Can you work these out from the model? Positions are in its coordinate system, mm. Give positions to 0.01 mm unless a question says otherwise; leave off trailing zeros. Loops run counter-clockwise (first coordinate to the right, second up) from the corner with the lowest first, then second, coordinate; pieces in that order, holes last. Notation, with made-up numbers: M 75,66.25 L 100,66.25 A20 ccw 100,96.25 Z; hole C -3,63.5 d9. An arc over 180 degrees is marked long. Put each result on its own line as item: value. Start each with the question number.
1) Imagine slicing it at A-A (z = -4). Write out the boundary of the cut face in (x, y).
2) Imagine slicing it at B-B (x = -11). Write out the boundary of the cut face in (y, z), then the cut area to 3 significant figures.
3) Please list where these lines run through material, in increasing order: line 1 along Z through (x, y) = (-44, 2); line 2 along X through (y, z) = (1.55, -50); line 3 along X through (y, z) = (1.35, -7.5). Write a range as from..to.
4) Imagine slicing it at C-C (y = 0.95). State how many separate pieces and enclosed holes the cut face has, then the cut area to 3 significant figures.
from build123d import *

# Parameters (mm, degrees)
SKETCH1_W           = 230
SKETCH1_H           = 103
BOSS_EXTRUDE1_DEPTH = 3
SKETCH2_W           = 85
SKETCH2_H           = 50.2
CUT_EXTRUDE1_DEPTH  = 3
SKETCH3_R           = 1.5
SKETCH3_W           = 31.00355617
SKETCH3_H           = 13
CUT_EXTRUDE2_DEPTH  = 3
SKETCH4_R           = 1
CUT_EXTRUDE3_DEPTH  = 3


with BuildPart() as part:
    # Sketch1 → Boss-Extrude1 (new body)
    with BuildSketch(Plane(origin=(0, 0, 0), x_dir=(1, 0, 0), z_dir=(0, 1, 0))):
        with Locations((2.626404494, 17.846910112)):
            Rectangle(SKETCH1_W, SKETCH1_H)
    extrude(amount=BOSS_EXTRUDE1_DEPTH)

    # Sketch2 → Cut-Extrude1 (cut)
    with BuildSketch(Plane(origin=(0, 3, 0), x_dir=(1, 0, 0), z_dir=(0, 1, 0))):
        with Locations((-39.873595506, 19.346910112)):
            Rectangle(SKETCH2_W, SKETCH2_H)
    extrude(amount=-CUT_EXTRUDE1_DEPTH, mode=Mode.SUBTRACT)

    # Sketch3 → Cut-Extrude2 (cut)
    with BuildSketch(Plane(origin=(0, 3, 0), x_dir=(1, 0, 0), z_dir=(0, 1, 0))):
        with Locations(Location((37.126404494, 49.846910112, 0), (0, 0, 270))):
            Circle(SKETCH3_R)
        with Locations(Location((88.126404494, 49.846910112, 0), (0, 0, 270))):
            Circle(SKETCH3_R)
        with Locations(Location((88.126404494, -11.153089888, 0), (0, 0, 270))):
            Circle(SKETCH3_R)
        with Locations(Location((37.126404494, -11.153089888, 0), (0, 0, 270))):
            Circle(SKETCH3_R)
        with Locations((62.624626409, -9.153089888)):
            Rectangle(SKETCH3_W, SKETCH3_H)
    extrude(amount=-CUT_EXTRUDE2_DEPTH, mode=Mode.SUBTRACT)

    # Sketch4 → Cut-Extrude3 (cut)
    with BuildSketch(Plane(origin=(0, 3, 0), x_dir=(1, 0, 0), z_dir=(0, 1, 0))):
        with Locations(Location((-83.873595506, 51.846910112, 0), (0, 0, 270))):
            Circle(SKETCH4_R)
        with Locations(Location((4.126404494, 51.846910112, 0), (0, 0, 270))):
            Circle(SKETCH4_R)
        with Locations(Location((-83.873595506, -13.153089888, 0), (0, 0, 270))):
            Circle(SKETCH4_R)
        with Locations(Location((4.126404494, -13.153089888, 0), (0, 0, 270))):
            Circle(SKETCH4_R)
    extrude(amount=-CUT_EXTRUDE3_DEPTH, mode=Mode.SUBTRACT)


solid = part.part
Recorded:
1. outline: M -112.37,0 L -82.37,0 L -82.37,3 L -112.37,3 Z; M 2.63,0 L 117.63,0 L 117.63,3 L 2.63,3 Z
2. outline: M 0,-69.35 L 3,-69.35 L 3,-44.45 L 0,-44.45 Z; M 0,5.75 L 3,5.75 L 3,33.65 L 0,33.65 Z
2. area: 158 mm²
3. line 1: -69.35..-44.45, 5.75..33.65
3. line 2: -112.37..35.63, 38.62..86.63, 89.62..117.63
3. line 3: -112.37..-82.37, 2.63..117.63
4. separate pieces: 1
4. enclosed holes: 10
4. area: 19,000 mm²
